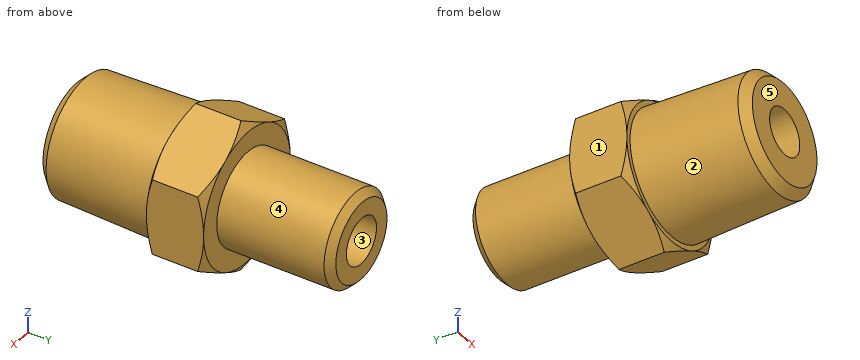
```python
from build123d import *

# Parameters (mm, degrees)
SKETCH7_R               = 5.1435
BOSS_EXTRUDE3_DEPTH     = 9.525
BOSS_EXTRUDE3_DRAFT     = -1.783333333
BOSS_EXTRUDE4_DEPTH     = 4.7625
SKETCH9_R               = 3.8735
BOSS_EXTRUDE5_DEPTH     = 9.525
SKETCH10_R              = 1.9304
CUT_EXTRUDE1_DEPTH      = 26.279826392
SKETCH11_OUTSIDE_W      = 79.992
SKETCH11_OUTSIDE_H      = 81.712
SKETCH11_OUTSIDE_R      = 5.55625
CUT_EXTRUDE2_DEPTH      = 17.618276758
CUT_EXTRUDE2_DRAFT      = 60
MIRROR1_COPY_1_SKETCH_W = 79.992
MIRROR1_COPY_1_SKETCH_H = 81.712
MIRROR1_COPY_1_SKETCH_R = 5.55625
MIRROR1_COPY_1_DEPTH    = 17.618276758
MIRROR1_COPY_1_DRAFT    = 60
CHAMFER1_SIZE           = 0.705555556
CHAMFER1_SIZE2          = 0.728581919
CHAMFER2_SIZE           = 0.5953125


with BuildPart() as part:
    # Sketch7 → Boss-Extrude3 (with draft: the straight prism first)
    with BuildSketch(Plane(origin=(0, 9.525, 0), x_dir=(1, 0, 0), z_dir=(0, 1, 0))):
        Circle(SKETCH7_R)
    extrude(amount=-BOSS_EXTRUDE3_DEPTH)
    # Boss-Extrude3: the draft: its side faces are tilted about the plane it starts from
    boss_extrude3_sides = [part.faces().sort_by_distance(p)[0] for p in [
        (-5.1435, 4.7625, 0),
    ]]
    draft(boss_extrude3_sides, Plane(origin=(0, 9.525, 0), x_dir=(1, 0, 0), z_dir=(0, 1, 0)), BOSS_EXTRUDE3_DRAFT)

    # Sketch8 → Boss-Extrude4 (add)
    with BuildSketch(Plane(origin=(0, 9.525, 0), x_dir=(1, 0, 0), z_dir=(0, 1, 0))):
        Polygon((5.55625, -3.207902433), (5.55625, 3.207902433), (0, 6.415804866), (-5.55625, 3.207902433), (-5.55625, -3.207902433), (0, -6.415804866), align=None)
    extrude(amount=BOSS_EXTRUDE4_DEPTH)

    # Sketch9 → Boss-Extrude5 (add)
    with BuildSketch(Plane(origin=(0, 23.8125, 0), x_dir=(1, 0, 0), z_dir=(0, 1, 0))):
        with Locations(Location((0, 0, 0), (0, 0, 270))):
            Circle(SKETCH9_R)
    extrude(amount=-BOSS_EXTRUDE5_DEPTH)

    # Sketch10 → Cut-Extrude1 (cut, through all)
    with BuildSketch(Plane(origin=(0, 0, 0), x_dir=(1, 0, 0), z_dir=(0, 1, 0))):
        with Locations(Location((0, 0, 0), (0, 0, 270))):
            Circle(SKETCH10_R)
    extrude(amount=CUT_EXTRUDE1_DEPTH, mode=Mode.SUBTRACT)


with BuildPart() as cut_extrude2_tool:
    # Sketch11 outside → Cut-Extrude2 (with draft: the straight prism first)
    with BuildSketch(Plane(origin=(0, 9.525, 0), x_dir=(1, 0, 0), z_dir=(0, 1, 0))):
        Rectangle(SKETCH11_OUTSIDE_W, SKETCH11_OUTSIDE_H)
        Circle(SKETCH11_OUTSIDE_R, mode=Mode.SUBTRACT)
    extrude(amount=CUT_EXTRUDE2_DEPTH)
    # Cut-Extrude2: the draft: its side faces are tilted about the plane it starts from
    cut_extrude2_sides = [cut_extrude2_tool.faces().sort_by_distance(p)[0] for p in [
        (0, 18.334138379, 40.856),
        (39.996, 18.334138379, 0),
        (0, 18.334138379, -40.856),
        (-39.996, 18.334138379, 0),
        (-5.55625, 18.334138379, 0),
    ]]
    draft(cut_extrude2_sides, Plane(origin=(0, 9.525, 0), x_dir=(1, 0, 0), z_dir=(0, 1, 0)), CUT_EXTRUDE2_DRAFT)


with BuildPart() as part_1:
    add(part.part)

    # Cut-Extrude2: cut by cut_extrude2_tool
    add(cut_extrude2_tool.part, mode=Mode.SUBTRACT)


with BuildPart() as mirror1_copy_1_tool:
    # Mirror1 copy 1 sketch → Mirror1 copy 1 (with draft: the straight prism first)
    with BuildSketch(Plane.XZ.offset(-14.2875)):
        Rectangle(MIRROR1_COPY_1_SKETCH_W, MIRROR1_COPY_1_SKETCH_H)
        Circle(MIRROR1_COPY_1_SKETCH_R, mode=Mode.SUBTRACT)
    extrude(amount=MIRROR1_COPY_1_DEPTH)
    # Mirror1 copy 1: the draft: its side faces are tilted about the plane it starts from
    mirror1_copy_1_sides = [mirror1_copy_1_tool.faces().sort_by_distance(p)[0] for p in [
        (0, 5.478361621, 40.856),
        (39.996, 5.478361621, 0),
        (0, 5.478361621, -40.856),
        (-39.996, 5.478361621, 0),
        (-5.55625, 5.478361621, 0),
    ]]
    draft(mirror1_copy_1_sides, Plane.XZ.offset(-14.2875), MIRROR1_COPY_1_DRAFT)


with BuildPart() as part_2:
    add(part_1.part)

    # Mirror1 copy 1: cut by mirror1_copy_1_tool
    add(mirror1_copy_1_tool.part, mode=Mode.SUBTRACT)

    # Chamfer1
    chamfer1_edges = [part_2.edges().sort_by_distance(p)[0] for p in [
        (-4.846938237, 0, 0),
    ]]
    chamfer1_side = [part_2.faces().sort_by_distance(p)[0] for p in [
        (-4.709846121, 0, 0),
    ]]
    chamfer(chamfer1_edges, length=CHAMFER1_SIZE, length2=CHAMFER1_SIZE2, reference=chamfer1_side[0])

    # Chamfer2
    chamfer2_edges = [part_2.edges().sort_by_distance(p)[0] for p in [
        (0, 23.8125, -3.8735),
    ]]
    chamfer(chamfer2_edges, length=CHAMFER2_SIZE)


solid = part_2.part
```
Check sheet for the modelled part. Datum: model origin and axes. Units: mm. Face numbers are marked on the shaded views. A direction names the side the tool comes from. Coordinates: 2 decimals unless noted, no trailing zeros. Loops run counter-clockwise (first coordinate to the right, second up) from the corner with the lowest first, then second, coordinate; pieces in that order, holes last.
1) Gauge pin test, flat ends, axial feed: pin 1 (1.5 mm diameter, centred on y = 14, z = -5, fed in from -X); pin 2 (6 mm diameter, centred on x = -3, y = 5.5, fed in from +Z); pin 3 (1 mm diameter, centred on x = 3.5, z = 4, fed in from +Y). Record the tip position at first contact, or that the pin passes through.
2) Sectioned sample at A-A (y = 19.75). Record the boundary of the cut face in (x, z), and give its area (3 significant figures).
3) Sectioned sample at B-B (y = 4.5). Record the boundary of the cut face in (x, z).
4) Material ranges on probe 1 along X at (y, z) = (15.75, 0); probe 2 along X at (y, z) = (12.25, 0); probe 3 along Z at (x, y) = (-0.75, 10.5), recorded low to high.
5) Access from +Z, -Z, +X, -X, +Y, -Y to the whole of each face (thin tool, end or side, straight path). Record for the marked faces 4 and 5.
6) Release check for a two-part mould opening along Z. For the marked faces 1, 2 and 3 record: released by +Z, released by -Z, zero draft, split by the parting line, or undercut.
Check sheet entries:
1. pin 1: stops at x = -3.75
1. pin 2: stops at z = 5.05
1. pin 3: stops at y = 14.29
2. outline: circle Ø7.75 at (0, 0); hole circle Ø3.86 at (0, 0)
2. area: 35.4 mm2
3. outline: circle Ø9.97 at (0, 0); hole circle Ø3.86 at (0, 0)
4. probe 1: x = -3.87 to -1.93, 1.93 to 3.87
4. probe 2: x = -5.56 to -1.93, 1.93 to 5.56
4. probe 3: z = -5.98 to -1.78, 1.78 to 5.98
5. face 4: +Y
5. face 5: +Z, -Z, +X, -X, -Y
6. face 1: zero draft
6. face 2: split by the parting line
6. face 3: undercut
